Design review of the part built by this model. Coordinates are the model's own, in mm. Face numbers are marked on the shaded views. Round coordinates to 2 decimals unless told otherwise and drop trailing zeros. Loops run counter-clockwise (first coordinate to the right, second up) from the corner with the lowest first, then second, coordinate; pieces in that order, holes last. Notation, with made-up numbers: (36.25, 53) - (48.25, 53) arc R16 ccw to (48.25, 73) - close; hole circle Ø2 at (28.5, 14). An arc over 180 degrees is marked (long way). Use one line per item in the form item = value. Start each with the question number.
(1) Wall thickness on probe 1 along Y at (x, z) = (-4, 0); probe 2 along Z at (x, y) = (-2, 0.9); probe 3 along X at (y, z) = (0.6, 2.5): over which ranges is each line inside the solid? List them lowest first. Write a range as [from, to].
(2) We need section B-B, the plane z = 0. Write out the cut boundary in (x, y).
(3) We need section A-A, the plane x = 0. Write out the cut boundary in (y, z), then the cut area to 3 significant figures.
(4) The part is to be moulded in two halves that separate along Z. For the marked faces 1 and 2, say which applies: released by +Z, released by -Z, zero draft, split by the parting line, or undercut.
(5) We need section C-C, the plane y = 1.4. Write out the cut boundary in (x, z).
(6) We need section D-D, the plane y = 2.05. Write out the cut boundary in (x, z), then the cut area to 3 significant figures.
(7) For pin 1 (4 mm diameter, centred on x = 0, z = 0, fed in from +Y); pin 2 (3 mm diameter, centred on x = -1.5, z = -3.5, fed in from +Y); pin 3 (2 mm diameter, centred on x = -3.5, y = 1.5, fed in from +Z); pin 4 (1 mm diameter, centred on y = 0.5, z = 3, fed in from +X), all flat-tipped, find the tip position at first contact; note any pin that passes through.
from build123d import *


with BuildPart() as part:
    # Sketch1 → Revolve1 (revolve)
    with BuildSketch(Plane.XY, mode=Mode.PRIVATE) as revolve1_sk:
        with BuildLine():
            Line((3, 0), (3, 4))
            ThreePointArc((3, 4), (4.472135955, 2.236067977), (5, 0))
            Line((5, 0), (3, 0))
        make_face()
    revolve(revolve1_sk.sketch.rotate(Axis((0, 0, 0), (0, 1, 0)), 90), axis=Axis((0, 0, 0), (0, 1, 0)))

    # Sketch2 → Cut-Revolve1 (revolve, cut)
    with BuildSketch(Plane(origin=(0, 0, 0), x_dir=(0, 0, -1), z_dir=(1, 0, 0))):
        Polygon((3.283055217, 3.771146834), (3.283055217, 3.53723963), (3.383055217, 3.53723963), (3.383055217, 3.783827608), (3.383055217, 3.915367926), (3.283055217, 3.915367926), align=None)
    revolve(axis=Axis((0, 0, 0), (0, 1, 0)), mode=Mode.SUBTRACT)


solid = part.part
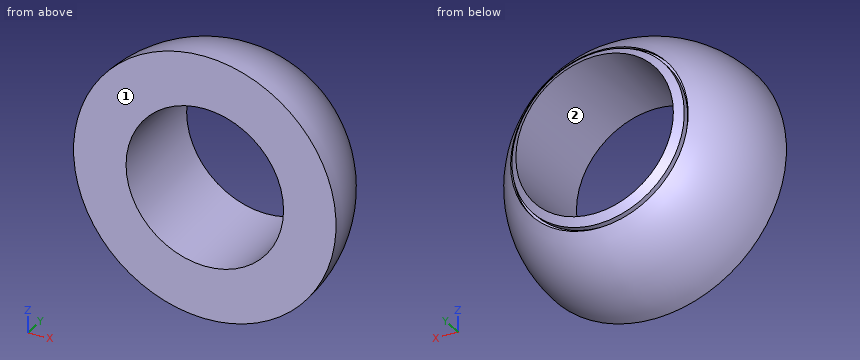
Data:
q1.probe_1 = [0, 3]
q1.probe_2 = [-4.49, -2.24], [2.24, 4.49]
q1.probe_3 = [-4.29, -1.66], [1.66, 4.29]
q2.outline = (-5, 0) - (-3, 0) - (-3, 4) arc R5 ccw to (-3.28, 3.77) - (-3.28, 3.54) - (-3.38, 3.54) - (-3.38, 3.68) arc R5 ccw to start; (3, 0) - (5, 0) arc R5 ccw to (3.38, 3.68) - (3.38, 3.54) - (3.28, 3.54) - (3.28, 3.77) arc R5 ccw to (3, 4) - close
q3.outline = (0, -5) arc R5 ccw to (3.68, -3.38) - (3.54, -3.38) - (3.54, -3.28) - (3.77, -3.28) arc R5 ccw to (4, -3) - (0, -3) - close; (0, 3) - (4, 3) arc R5 ccw to (3.77, 3.28) - (3.54, 3.28) - (3.54, 3.38) - (3.68, 3.38) arc R5 ccw to (0, 5) - close
q3.area = 11.1 mm^2
q4.face_1 = zero draft
q4.face_2 = undercut
q5.outline = circle Ø9.6 at (0, 0); hole circle Ø6 at (0, 0)
q6.outline = circle Ø9.12 at (0, 0); hole circle Ø6 at (0, 0)
q6.area = 37.1 mm^2
q7.pin_1 = through
q7.pin_2 = 4
q7.pin_3 = 4.14
q7.pin_4 = 4.31
